from build123d import *

# Parameters (mm, degrees)
BOSS_EXTRU_1_DEPTH = 5


with BuildPart() as part:
    # Esquisse1 → Boss.-Extru.1 (new body)
    with BuildSketch(Plane.XY):
        Polygon((82.539833849, -153.626771729), (18.539833849, -153.626771729), (18.539833849, -152.626771729), (15.539833849, -152.626771729), (15.539833849, -153.626771729), (8.539833849, -153.626771729), (-6.460166151, -127.646009615), (-6.460166151, -120.646009615), (-5.460166151, -120.646009615), (-5.460166151, -117.646009615), (-6.460166151, -117.646009615), (-6.460166151, -106.469095079), (-5.460166151, -106.469095079), (-5.460166151, -103.469095079), (-6.460166151, -103.469095079), (-6.460166151, -96.469095079), (8.539833849, -70.488332966), (15.539833849, -70.488332966), (15.539833849, -71.488332966), (18.539833849, -71.488332966), (18.539833849, -70.488332966), (82.539833849, -70.488332966), (82.539833849, -71.488332966), (85.539833849, -71.488332966), (85.539833849, -70.488332966), (92.539833849, -70.488332965), (107.539833849, -96.469095079), (107.539833849, -103.469095079), (106.539833849, -103.469095079), (106.539833849, -106.469095079), (107.539833849, -106.469095079), (107.539833849, -117.646009615), (106.539833849, -117.646009615), (106.539833849, -120.646009615), (107.539833849, -120.646009615), (107.539833849, -127.646009615), (92.539833849, -153.626771729), (85.539833849, -153.626771729), (85.539833849, -152.626771729), (82.539833849, -152.626771729), align=None)
        Polygon((0.539833849, -106.469095079), (0.539833849, -117.646009615), (-0.460166151, -117.646009615), (-0.460166151, -120.646009615), (0.539833849, -120.646009615), (0.539833849, -125.770365268), (12.581285733, -146.626771729), (15.539833849, -146.626771729), (15.539833849, -147.626771729), (18.539833849, -147.626771729), (18.539833849, -146.626771729), (82.539833849, -146.626771729), (82.539833849, -147.626771729), (85.539833849, -147.626771729), (85.539833849, -146.626771729), (88.498381965, -146.626771729), (100.539833849, -125.770365268), (100.539833849, -120.646009615), (101.539833849, -120.646009615), (101.539833849, -117.646009615), (100.539833849, -117.646009615), (100.539833849, -106.469095079), (101.539833849, -106.469095079), (101.539833849, -103.469095079), (100.539833849, -103.469095079), (0.539833849, -103.469095079), (-0.460166151, -103.469095079), (-0.460166151, -106.469095079), align=None, mode=Mode.SUBTRACT)
        Polygon((18.539833849, -77.488332966), (82.539833849, -77.488332966), (82.539833849, -76.488332966), (85.539833849, -76.488332966), (85.539833849, -77.488332966), (88.498381965, -77.488332966), (89.641975504, -79.469095079), (11.437692194, -79.469095079), (12.581285733, -77.488332966), (15.539833849, -77.488332966), (15.539833849, -76.488332966), (18.539833849, -76.488332966), align=None, mode=Mode.SUBTRACT)
    extrude(amount=BOSS_EXTRU_1_DEPTH)


solid = part.part
Source: CAD feature listing. Evaluate the final solid. Frame: model axes, mm. A direction names the side the tool comes from. Give positions to 0.01 mm unless a question says otherwise; leave off trailing zeros. Write each loop counter-clockwise with the first axis right and the second up, starting at its lowest first coordinate (ties: lowest second). Pieces come first, ordered by that corner, then holes. Notation, with made-up numbers: M -25.75,-32.75 L 5.25,-32.75 A27 ccw 5.25,-14.75 Z; hole C 17,-11 d8. An arc over 180 degrees is marked long. Return JSON: item names as keys, results as strings. Group by question number.
1) Cut plane D-D, the plane x = 17. Output: boundary loops of the cut face in (y, z).
2) Cut plane A-A, the plane y = -111. Output: boundary loops of the cut face in (x, z).
3) First-contact query: pin 1 Ø0.5 at (y, z) = (-77, 3) entering from -X; pin 2 Ø0.5 at (y, z) = (-153, 2.5) entering from +X; pin 3 Ø2 at (x, y) = (20, -82) entering from -Z; pin 4 Ø0.5 at (x, z) = (-6, 1.5) entering from -Y. Flat tips, straight axial feed; report the tip coordinate or a pass-through.
4) Ray query, L1, parallel to Y at x = 80.5, z = 0.5; L2, parallel to Y at x = 83, z = 4.7; L3, parallel to X at y = -106, z = 0.5. Return the intervals inside material, ascending.
5) Set-up query: faces 1 (the face through (84, -71.488, 2)), 2 (the face through (-5.46, -119, 2)), 3 (the face through (50, -103.469, 2)), 4 (the face through (106.54, -119, 2)). Return all of +Z, -Z, +X, -X, +Y, -Y with unobstructed straight access to the full face (end or side cutting, diameter ignored); none if empty.
6) Cut plane C-C, the plane x = 2. Output: boundary loops of the cut face in (y, z).
7) Draft query along X for faces 5 (the face through (-6.46, -124, 2)), 6 (the face through (51, -153.627, 2)), 7 (the face through (84, -147.627, 2)), 8 (the face through (50, -146.627, 2)). Return one class per face: released by +X, released by -X, zero draft, split by the parting line, or undercut.
8) Cut plane B-B, the plane x = 50. Output: boundary loops of the cut face in (y, z), then the cut area to 3 significant figures.
Data:
{
 "1": {"outline": "M -152.63,0 L -147.63,0 L -147.63,5 L -152.63,5 Z; M -103.47,0 L -79.47,0 L -79.47,5 L -103.47,5 Z; M -76.49,0 L -71.49,0 L -71.49,5 L -76.49,5 Z"},
 "2": {"outline": "M -6.46,0 L 0.54,0 L 0.54,5 L -6.46,5 Z; M 100.54,0 L 107.54,0 L 107.54,5 L 100.54,5 Z"},
 "3": {"pin 1": "stops at x = 4.64", "pin 2": "stops at x = 93.05", "pin 3": "stops at z = 0", "pin 4": "stops at y = -128.88"},
 "4": {"L1": "y = -153.63 to -146.63, -103.47 to -79.47, -77.49 to -70.49", "L2": "y = -152.63 to -147.63, -103.47 to -79.47, -76.49 to -71.49", "L3": "x = -5.46 to -0.46, 101.54 to 106.54"},
 "5": {"face 1": "+Z, -Z, +Y", "face 2": "+Z, -Z, -X", "face 3": "+Z, -Z", "face 4": "+Z, -Z, +X"},
 "6": {"outline": "M -142.3,0 L -128.3,0 L -128.3,5 L -142.3,5 Z; M -103.47,0 L -81.82,0 L -81.82,5 L -103.47,5 Z"},
 "7": {"face 5": "released by -X", "face 6": "zero draft", "face 7": "undercut", "face 8": "undercut"},
 "8": {"outline": "M -153.63,0 L -146.63,0 L -146.63,5 L -153.63,5 Z; M -103.47,0 L -79.47,0 L -79.47,5 L -103.47,5 Z; M -77.49,0 L -70.49,0 L -70.49,5 L -77.49,5 Z", "area": "190 mm²"}
}
